from build123d import *
from OCP.BRepFilletAPI import BRepFilletAPI_MakeChamfer

# Parameters (mm, degrees)
SKETCH_1_W                  = 150
SKETCH_1_H                  = 85
EXTRUDE_1_DEPTH             = 2
SKETCH_1_2_W                = 150
SKETCH_1_2_H                = 85
SKETCH_1_2_W_2              = 144
SKETCH_1_2_H_2              = 79
EXTRUDE_1_2_DEPTH           = 15
SKETCH_4_R                  = 2.25
EXTRUDE_2_DEPTH             = 3
CUT_EXTRUDE_2_REACH         = 92.04
SKETCH_6_R                  = 1.75
SKETCH_10_W                 = 1
SKETCH_10_H                 = 1
SKETCH_10_W_2               = 7
SKETCH_10_H_2               = 7
EXTRUDE_4_DEPTH             = 20
CHAMFER_1_SIZE              = 15
CHAMFER_1_SIZE2             = 4.019237886
SKETCH_13_R                 = 3
SKETCH_13_R_2               = 2.25
EXTRUDE_5_DEPTH             = 0.5
CHAMFER_1_OF_MIRROR_2_SIZE  = 15
CHAMFER_1_OF_MIRROR_2_SIZE2 = 4.019237886
SKETCH_12_R                 = 2.55
HOLE_WIZARD_M2_1_D          = 1.6


with BuildPart() as part:
    # 草圖1 → Extrude 1 (new body)
    with BuildSketch(Plane(origin=(0, 0, 0), x_dir=(1, 0, 0), z_dir=(0, 1, 0))):
        Rectangle(SKETCH_1_W, SKETCH_1_H)
    extrude(amount=-EXTRUDE_1_DEPTH)

    # 草圖1<2> → Extrude 1 2 (add)
    with BuildSketch(Plane(origin=(0, 0, 0), x_dir=(1, 0, 0), z_dir=(0, 1, 0))):
        Rectangle(SKETCH_1_2_W, SKETCH_1_2_H)
        Rectangle(SKETCH_1_2_W_2, SKETCH_1_2_H_2, mode=Mode.SUBTRACT)
    extrude(amount=-EXTRUDE_1_2_DEPTH)

    # 草圖4 → 填料-伸長2 (add)
    # profile 1 of 2: a face of its own
    with BuildSketch(Plane.XY.offset(42.5)):
        with BuildLine():
            Line((-75, -15), (-72.846954236, -23.03527618))
            ThreePointArc((-72.846954236, -23.03527618), (-68.983250931, -26), (-65.119547626, -23.03527618))
            Line((-65.119547626, -23.03527618), (-62.966501863, -15))
            Line((-62.966501863, -15), (-75, -15))
        make_face()
        with Locations(Location((-68.983250931, -22, 0), (0, 0, 180))):
            Circle(SKETCH_4_R, mode=Mode.SUBTRACT)
    # profile 2 of 2: a face of its own
    with BuildSketch(Plane.XY.offset(42.5)):
        with BuildLine():
            Line((62.966501863, -15), (75, -15))
            Line((75, -15), (72.846954236, -23.03527618))
            ThreePointArc((72.846954236, -23.03527618), (68.983250931, -26), (65.119547626, -23.03527618))
            Line((65.119547626, -23.03527618), (62.966501863, -15))
        make_face()
        with Locations((68.983250931, -22)):
            Circle(SKETCH_4_R, mode=Mode.SUBTRACT)
    extrude_2 = extrude(amount=-EXTRUDE_2_DEPTH)

    # 鏡射1: 填料-伸長2 across plane
    add(extrude_2.mirror(Plane.XY))

    # 草圖6 → 除料-伸長2 (cut, up to next)
    with BuildSketch(Plane(origin=(0, 0, 0), x_dir=(1, 0, 0), z_dir=(0, 1, 0)), mode=Mode.PRIVATE) as cut_extrude_2_sk1:
        with Locations(Location((-38.5, -36.5, 0), (0, 0, 270))):
            Circle(SKETCH_6_R)
    cut_extrude_2_tool1 = extrude(cut_extrude_2_sk1.sketch, amount=-CUT_EXTRUDE_2_REACH, mode=Mode.PRIVATE) & part.part
    # 草圖6 → 除料-伸長2 (cut, up to next)
    with BuildSketch(Plane(origin=(0, 0, 0), x_dir=(1, 0, 0), z_dir=(0, 1, 0)), mode=Mode.PRIVATE) as cut_extrude_2_sk2:
        with Locations(Location((38.5, -36.5, 0), (0, 0, 270))):
            Circle(SKETCH_6_R)
    cut_extrude_2_tool2 = extrude(cut_extrude_2_sk2.sketch, amount=-CUT_EXTRUDE_2_REACH, mode=Mode.PRIVATE) & part.part
    # 草圖6 → 除料-伸長2 (cut, up to next)
    with BuildSketch(Plane(origin=(0, 0, 0), x_dir=(1, 0, 0), z_dir=(0, 1, 0)), mode=Mode.PRIVATE) as cut_extrude_2_sk3:
        with Locations(Location((38.5, 36.5, 0), (0, 0, 270))):
            Circle(SKETCH_6_R)
    cut_extrude_2_tool3 = extrude(cut_extrude_2_sk3.sketch, amount=-CUT_EXTRUDE_2_REACH, mode=Mode.PRIVATE) & part.part
    # 草圖6 → 除料-伸長2 (cut, up to next)
    with BuildSketch(Plane(origin=(0, 0, 0), x_dir=(1, 0, 0), z_dir=(0, 1, 0)), mode=Mode.PRIVATE) as cut_extrude_2_sk4:
        with Locations(Location((-38.5, 36.5, 0), (0, 0, 270))):
            Circle(SKETCH_6_R)
    cut_extrude_2_tool4 = extrude(cut_extrude_2_sk4.sketch, amount=-CUT_EXTRUDE_2_REACH, mode=Mode.PRIVATE) & part.part
    add(cut_extrude_2_tool1.solids().sort_by_distance((-38.5, 0, 36.5))[0], mode=Mode.SUBTRACT)
    add(cut_extrude_2_tool2.solids().sort_by_distance((38.5, 0, 36.5))[0], mode=Mode.SUBTRACT)
    add(cut_extrude_2_tool3.solids().sort_by_distance((38.5, 0, -36.5))[0], mode=Mode.SUBTRACT)
    add(cut_extrude_2_tool4.solids().sort_by_distance((-38.5, 0, -36.5))[0], mode=Mode.SUBTRACT)

    # 草圖10 → 填料-伸長4 (add)
    with BuildSketch(Plane(origin=(0, 0, 0), x_dir=(1, 0, 0), z_dir=(0, 1, 0))):
        with Locations((-74.5, -42)):
            Rectangle(SKETCH_10_W, SKETCH_10_H)
        with Locations((-70.5, -42)):
            Rectangle(SKETCH_10_W_2, SKETCH_10_H)
        with Locations((-74.5, -38)):
            Rectangle(SKETCH_10_W, SKETCH_10_H_2)
    extrude_4 = extrude(amount=EXTRUDE_4_DEPTH)

    # 導角1: one chamfer whose edges measure the first distance from different faces: ONE call of the kernel's chamfer builder (chamfer() names one face for all edges)
    chamfer_1_edges_1 = [part.edges().sort_by_distance(p)[0] for p in [
        (-67, 20, 42),
    ]]
    chamfer_1_side_1 = [part.faces().sort_by_distance(p)[0] for p in [
        (-67, 10, 42),
    ]]
    chamfer_1_edges_2 = [part.edges().sort_by_distance(p)[0] for p in [
        (-74.5, 20, 34.5),
    ]]
    chamfer_1_side_2 = [part.faces().sort_by_distance(p)[0] for p in [
        (-74.5, 10, 34.5),
    ]]
    chamfer_1 = BRepFilletAPI_MakeChamfer(part.part.solid().wrapped)
    for e in chamfer_1_edges_1:
        chamfer_1.Add(CHAMFER_1_SIZE, CHAMFER_1_SIZE2, e.wrapped, chamfer_1_side_1[0].wrapped)  # the first distance lies on this face
    for e in chamfer_1_edges_2:
        chamfer_1.Add(CHAMFER_1_SIZE, CHAMFER_1_SIZE2, e.wrapped, chamfer_1_side_2[0].wrapped)  # the first distance lies on this face
    add(Compound.cast(chamfer_1.Shape()), mode=Mode.REPLACE)

    # 草圖13 → 填料-伸長5 (add)
    # profile 1 of 2: a face of its own
    with BuildSketch(Plane.XY.offset(42.5)):
        with Locations((68.983250931, -22)):
            Circle(SKETCH_13_R)
        with Locations((68.983250931, -22)):
            Circle(SKETCH_13_R_2, mode=Mode.SUBTRACT)
    # profile 2 of 2: a face of its own
    with BuildSketch(Plane.XY.offset(42.5)):
        with Locations(Location((-68.983250931, -22, 0), (0, 0, 180))):
            Circle(SKETCH_13_R)
        with Locations(Location((-68.983250931, -22, 0), (0, 0, 180))):
            Circle(SKETCH_13_R_2, mode=Mode.SUBTRACT)
    extrude_5 = extrude(amount=EXTRUDE_5_DEPTH)

    # 鏡射2: 填料-伸長4, 填料-伸長5 across plane
    add(extrude_4.mirror(Plane.XY))
    add(extrude_5.mirror(Plane.XY))

    # 導角1 of 鏡射2: one chamfer whose edges measure the first distance from different faces: ONE call of the kernel's chamfer builder (chamfer() names one face for all edges)
    chamfer_1_of_mirror_2_edges_1 = [part.edges().sort_by_distance(p)[0] for p in [
        (-67, 20, -42),
    ]]
    chamfer_1_of_mirror_2_side_1 = [part.faces().sort_by_distance(p)[0] for p in [
        (-67, 10, -42),
    ]]
    chamfer_1_of_mirror_2_edges_2 = [part.edges().sort_by_distance(p)[0] for p in [
        (-74.5, 20, -34.5),
    ]]
    chamfer_1_of_mirror_2_side_2 = [part.faces().sort_by_distance(p)[0] for p in [
        (-74.5, 10, -34.5),
    ]]
    chamfer_1_of_mirror_2 = BRepFilletAPI_MakeChamfer(part.part.solid().wrapped)
    for e in chamfer_1_of_mirror_2_edges_1:
        chamfer_1_of_mirror_2.Add(CHAMFER_1_OF_MIRROR_2_SIZE, CHAMFER_1_OF_MIRROR_2_SIZE2, e.wrapped, chamfer_1_of_mirror_2_side_1[0].wrapped)  # the first distance lies on this face
    for e in chamfer_1_of_mirror_2_edges_2:
        chamfer_1_of_mirror_2.Add(CHAMFER_1_OF_MIRROR_2_SIZE, CHAMFER_1_OF_MIRROR_2_SIZE2, e.wrapped, chamfer_1_of_mirror_2_side_2[0].wrapped)  # the first distance lies on this face
    add(Compound.cast(chamfer_1_of_mirror_2.Shape()), mode=Mode.REPLACE)

    # 掃出17: sweep along a curve in space
    with BuildLine() as sweep_17_path:
        Line((-71.5, 0, 39), (-71.5, 41.886116992, 39))
        ThreePointArc((-71.5, 41.886116992, 39), (-72.145627118, 49.895229142, 39), (-74.065835097, 57.697505292, 39))
        Line((-83.33772234, 85.513167019, 39), (-74.065835097, 57.697505292, 39))
        ThreePointArc((-86.5, 95, 29), (-85.573790317, 92.221370952, 36.071067812), (-83.33772234, 85.513167019, 39))
        Line((-86.5, 95, 29), (-86.5, 95, -29))
        ThreePointArc((-86.5, 95, -29), (-85.573790317, 92.221370952, -36.071067812), (-83.33772234, 85.513167019, -39))
        Line((-83.33772234, 85.513167019, -39), (-74.065835097, 57.697505292, -39))
        ThreePointArc((-71.5, 41.886116992, -39), (-72.145627118, 49.895229142, -39), (-74.065835097, 57.697505292, -39))
        Line((-71.5, 41.886116992, -39), (-71.5, 0, -39))
    # 草圖12 → 掃出17 (sweep)
    with BuildSketch(Plane(origin=(0, 0, 0), x_dir=(1, 0, 0), z_dir=(0, 1, 0))):
        with Locations((-71.5, 39)):
            Circle(SKETCH_12_R)
    sweep(path=sweep_17_path.line)

    # M2 螺紋孔1 (through all)
    with Locations(Plane(origin=(0, 0, 0), x_dir=(1, 0, 0), z_dir=(0, 1, 0))):
        with Locations((-29, 17), (-15.6, 17), (-15.6, 9), (-29, 9)):
            Hole(HOLE_WIZARD_M2_1_D / 2)


solid = part.part
Geometry check sheet. Reference: the model listing, model coordinates, mm. A direction names the side the tool comes from. Give positions to 0.01 mm unless a question says otherwise; leave off trailing zeros. Loops run counter-clockwise (first coordinate to the right, second up) from the corner with the lowest first, then second, coordinate; pieces in that order, holes last. Notation, with made-up numbers: M -22.75,-37.75 L 33.25,-37.75 A29 ccw 33.25,-1.75 Z; hole C 66.5,-25 d1. An arc over 180 degrees is marked long. Write each question's results on one line, items separated by ' | '.
1) Section check A-A, the plane y = 14. Record the boundary of the cut face in (x, z), plus the area to 3 significant figures.
Answers follow:
outline: M -75,-42.5 L -69.41,-42.5 L -69.41,-41.5 L -71,-41.5 A2.55 ccw long -74,-38.5 L -74,-36.91 L -75,-36.91 Z; M -75,36.91 L -74,36.91 L -74,38.5 A2.55 ccw long -71,41.5 L -69.41,41.5 L -69.41,42.5 L -75,42.5 Z; hole M -74,-41.5 L -72,-41.5 A2.55 cw -74,-39.5 Z; hole M -74,39.5 A2.55 cw -72,41.5 L -74,41.5 Z | area: 61.1 mm2
2) Gauge pin test, flat ends, axial feed: pin 1 (3 mm diameter, centred on y = 10.5, z = -36, fed in from +X); pin 2 (1.6 mm diameter, centred on y = 5.5, z = 40, fed in from +X); pin 3 (1 mm diameter, centred on x = -59.5, z = -5, fed in from -Y); pin 4 (2.5 mm diameter, centred on x = -68.98, y = -22, fed in from -Z). Record the tip position at first contact, or that the pin passes through.
Answers follow:
pin 1: x = -69.44 | pin 2: x = -68.96 | pin 3: y = -2 | pin 4: through
3) Thickness scan on line 1 (Z direction, x = -15.6, y = -0.95); line 2 (X direction, y = -0.65, z = -9); line 3 (Z direction, x = 38, y = -1). Record the ranges inside material, lowest first.
Answers follow:
line 1: -42.5 to -17.8, -16.2 to -9.8, -8.2 to 42.5 | line 2: -75 to -29.8, -28.2 to -16.4, -14.8 to 75 | line 3: -42.5 to -38.18, -34.82 to 34.82, 38.18 to 42.5
4) Release check for a two-part mould opening along Z. For faces 6 (the face through (-1, -8, 42.5)), 7 (the face through (37.83, -0.986, -34.883)), 8 (the face through (70.021, -23.996, 41.226)) record: +Z half, -Z half, draft (parallel to the pull), parting line (faces both ways), or undercut.
Answers follow:
face 6: +Z half | face 7: undercut | face 8: draft
5) Section check B-B, the plane z = 12. Record the boundary of the cut face in (x, y), plus the area to 3 significant figures.
Answers follow:
outline: C -86.5,95 d5.1; M -75,-15 L -72,-15 L -72,-2 L 72,-2 L 72,-15 L 75,-15 L 75,0 L -75,0 Z | area: 398 mm2
6) Tool access check on faces 1 (the face through (-65.986, -22.132, -42.746)), 2 (the face through (-72, -8, 1)), 3 (the face through (-75, -6, 1)), 4 (the face through (-69.07, 20.65, -38.23)), 5 (the face through (-65.986, -22.132, 42.746)). Record the directions out of +Z, -Z, +X, -X, +Y, -Y that give a thin tool (end or side, any length) a straight path to the whole face; none if there is none.
Answers follow:
face 1: -Z | face 2: -Y | face 3: +Z, -Z, -X, -Y | face 4: none | face 5: +Z
7) Section check D-D, the plane y = 29. Record the boundary of the cut face in (x, z), plus the area to 3 significant figures.
Answers follow:
outline: C -71.5,-39 d5.1; C -71.5,39 d5.1 | area: 40.9 mm2
8) Section check C-C, the plane x = 60. Record the boundary of the cut face in (y, z).
Answers follow:
outline: M -15,-42.5 L 0,-42.5 L 0,42.5 L -15,42.5 L -15,39.5 L -2,39.5 L -2,-39.5 L -15,-39.5 Z
